Here's the drawing with two shaded views (mm, measured from the low corner). I have some questions. Round coordinates to 2 decimals unless told otherwise and drop trailing zeros. Order: outer loops, then holes, each group sorted by start corner. A loop starts at its lowest first (then second) coordinate and runs counter-clockwise, first axis right, second up.
Q1. If we section it at C-C (z = 34.5): Please give me the cut outline in (x, y), plus the area to 3 significant figures.
Q2. We'd pull the mould along X, two halves only. Please class the marked faces 1, 2, 3 and 4: pulls with the +X half, pulls with the -X half, needs draft (parallel to the pull), parting line crosses it, or undercut.
Q3. If we section it at D-D (z = 100.5): Please give me the cut outline in (x, y) (3 decimals).
Q4. Will these pins go through, and if not, where does the flat tip stop? P1, Ø1.5, axis at x = 59.5, y = 36, coming from the -Z side; P2, Ø1.5, axis at y = 68, z = 59, coming from the -X side; P3, Ø8, axis at x = 26, z = 80.5, coming from the -Y side; P4, Ø2, axis at y = 26.5, z = 27, coming from the -X side.
Q5. If I drill on line 1 (Y direction, x = 38.1, z = 97) (3 decimals); line 2 (X direction, y = 38, z = 80); line 3 (Y direction, x = 52.5, z = 115.5), over which ranges is the centre line in solid material (lowest first)?
Q6. If we section it at A-A (x = 38.1): Please give me the cut outline in (y, z) (3 decimals).
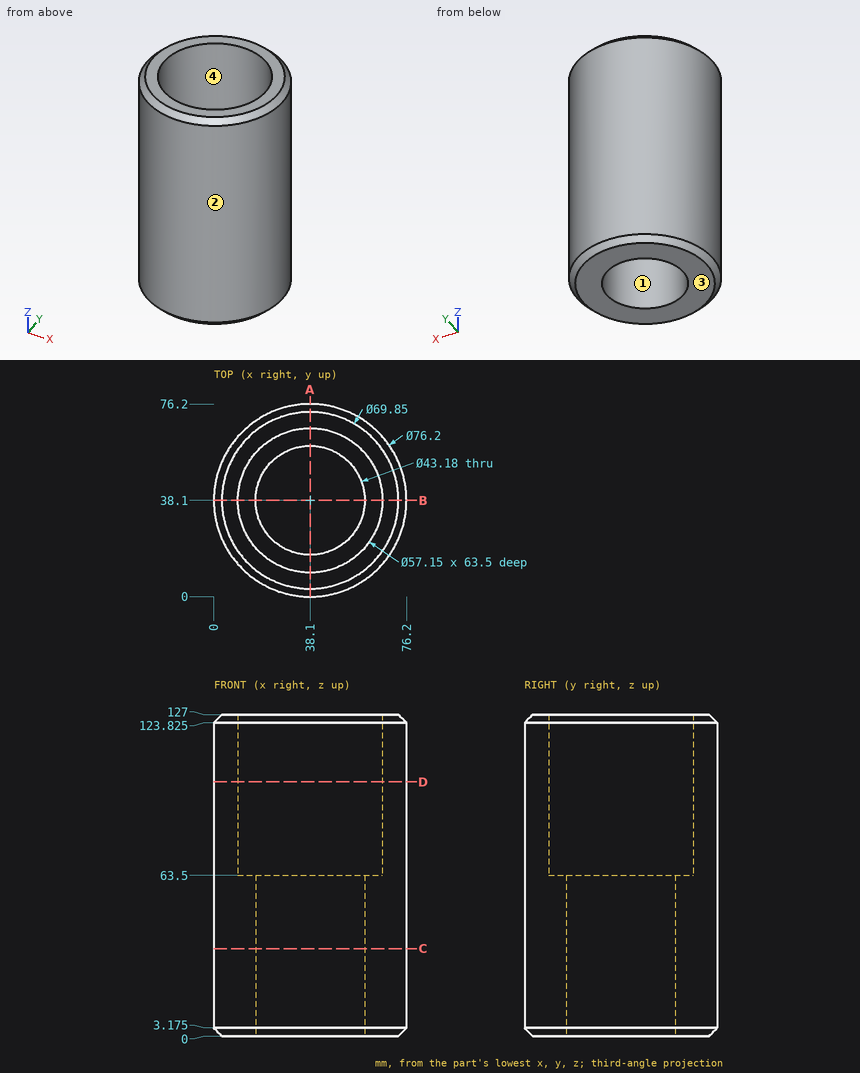
Solution:
1. outline: circle Ø76.2 at (38.1, 38.1); hole circle Ø43.18 at (38.1, 38.1)
1. area: 3,100 mm2
2. face 1: undercut
2. face 2: parting line crosses it
2. face 3: needs draft
2. face 4: undercut
3. outline: circle Ø76.2 at (38.1, 38.1); hole circle Ø57.15 at (38.1, 38.1)
4. P1: stops at z = 0
4. P2: stops at x = 13.57
4. P3: stops at y = 0.87
4. P4: stops at x = 1.5
5. line 1: y = 0 to 9.525, 66.675 to 76.2
5. line 2: x = 0 to 9.53, 66.67 to 76.2
5. line 3: y = 2.83 to 13.42, 62.78 to 73.37
6. outline: (0, 3.175) - (3.175, 0) - (16.51, 0) - (16.51, 63.5) - (9.525, 63.5) - (9.525, 127) - (3.175, 127) - (0, 123.825) - close; (59.69, 0) - (73.025, 0) - (76.2, 3.175) - (76.2, 123.825) - (73.025, 127) - (66.675, 127) - (66.675, 63.5) - (59.69, 63.5) - close
